from build123d import *

# Parameters (mm, degrees)
SZKIC1_R                    = 10.570763761
SZKIC1_R_2                  = 3
SZKIC1_R_3                  = 4
SZKIC1_R_4                  = 1
DODANIE_WYCI_GNI_CIE1_DEPTH = 5
SZKIC1_3_R                  = 10.570763761
SZKIC1_3_R_2                = 4
SZKIC1_3_R_3                = 1
DODANIE_WYCI_GNI_CIE2_DEPTH = 10


with BuildPart() as part:
    # Szkic1 → Dodanie-wyci_gni_cie1 (new body)
    with BuildSketch(Plane.XY):
        with BuildLine():
            Line((-50.67287635, -5.055665151), (-9.235111676, -10.570763761))
            ThreePointArc((-9.235111676, -10.570763761), (0, -11.182632843), (9.235111676, -10.570763761))
            Line((9.235111676, -10.570763761), (50.67287635, -5.055665151))
            ThreePointArc((50.67287635, -5.055665151), (55.100246338, 0), (50.67287635, 5.055665151))
            Line((50.67287635, 5.055665151), (9.235111676, 10.570763761))
            ThreePointArc((9.235111676, 10.570763761), (0, 11.182632843), (-9.235111676, 10.570763761))
            Line((-9.235111676, 10.570763761), (-50.67287635, 5.055665151))
            ThreePointArc((-50.67287635, 5.055665151), (-55.100246338, 0), (-50.67287635, -5.055665151))
        make_face()
        Circle(SZKIC1_R, mode=Mode.SUBTRACT)
        with Locations((50, 0)):
            Circle(SZKIC1_R_2, mode=Mode.SUBTRACT)
        with Locations((-50, 0)):
            Circle(SZKIC1_R_2, mode=Mode.SUBTRACT)
        Circle(SZKIC1_R)
        Circle(SZKIC1_R_3, mode=Mode.SUBTRACT)
        with Locations((-5.656854249, 5.656854249)):
            Circle(SZKIC1_R_4, mode=Mode.SUBTRACT)
        with Locations((-8, 0)):
            Circle(SZKIC1_R_4, mode=Mode.SUBTRACT)
        with Locations((0, 8)):
            Circle(SZKIC1_R_4, mode=Mode.SUBTRACT)
        with Locations((5.656854249, 5.656854249)):
            Circle(SZKIC1_R_4, mode=Mode.SUBTRACT)
        with Locations((8, 0)):
            Circle(SZKIC1_R_4, mode=Mode.SUBTRACT)
        with Locations((5.656854249, -5.656854249)):
            Circle(SZKIC1_R_4, mode=Mode.SUBTRACT)
        with Locations((0, -8)):
            Circle(SZKIC1_R_4, mode=Mode.SUBTRACT)
        with Locations((-5.656854249, -5.656854249)):
            Circle(SZKIC1_R_4, mode=Mode.SUBTRACT)
    extrude(amount=DODANIE_WYCI_GNI_CIE1_DEPTH)

    # Szkic1_3 → Dodanie-wyci_gni_cie2 (add)
    with BuildSketch(Plane.XY):
        Circle(SZKIC1_3_R)
        Circle(SZKIC1_3_R_2, mode=Mode.SUBTRACT)
        with Locations((-5.656854249, 5.656854249)):
            Circle(SZKIC1_3_R_3, mode=Mode.SUBTRACT)
        with Locations((-8, 0)):
            Circle(SZKIC1_3_R_3, mode=Mode.SUBTRACT)
        with Locations((0, 8)):
            Circle(SZKIC1_3_R_3, mode=Mode.SUBTRACT)
        with Locations((5.656854249, 5.656854249)):
            Circle(SZKIC1_3_R_3, mode=Mode.SUBTRACT)
        with Locations((8, 0)):
            Circle(SZKIC1_3_R_3, mode=Mode.SUBTRACT)
        with Locations((5.656854249, -5.656854249)):
            Circle(SZKIC1_3_R_3, mode=Mode.SUBTRACT)
        with Locations((0, -8)):
            Circle(SZKIC1_3_R_3, mode=Mode.SUBTRACT)
        with Locations((-5.656854249, -5.656854249)):
            Circle(SZKIC1_3_R_3, mode=Mode.SUBTRACT)
    extrude(amount=DODANIE_WYCI_GNI_CIE2_DEPTH)


solid = part.part
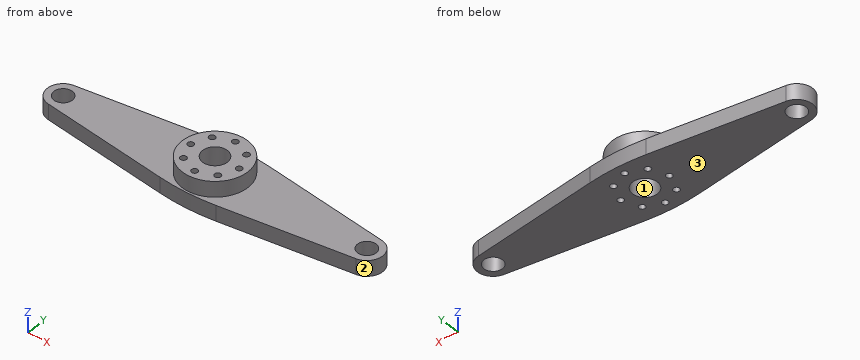
Geometry check sheet. Reference: the model listing, model coordinates, mm. Face numbers are marked on the shaded views. Round coordinates to 2 decimals unless told otherwise and drop trailing zeros. Order: outer loops, then holes, each group sorted by start corner. A loop starts at its lowest first (then second) coordinate and runs counter-clockwise, first axis right, second up. Notation, with made-up numbers: M 88,2 L 109,2 A27 cw 109,20 Z; hole C 19.5,-39 d11. An arc over 180 degrees is marked long. Write each question's results on one line, items separated by ' | '. Start each with the question number.
1. Cross-section at C-C on z = 6. Give the number of separate pieces and of enclosed holes in the cut face, plus the area to 3 significant figures.
2. Go/stop test with flat-tipped pins: P1, Ø10, axis at x = 26.5, y = -6.5, coming from the +Z side; P2, Ø6.5, axis at x = 0, y = 0, coming from the -Z side; P3, Ø2, axis at y = -2.5, z = 2, coming from the +X side; P4, Ø4, axis at y = 5, z = 8.5, coming from the +X side. Record where each tip stops, or that it passes through.
3. Draft check along X on the marked faces 1, 2 and 3. Enter one of: pulls with the +X half, pulls with the -X half, needs draft (parallel to the pull), parting line crosses it, or undercut.
4. Cross-section at B-B on y = -8. Record the boundary of the cut face in (x, z).
5. Cross-section at A-A on x = 0. Record the boundary of the cut face in (y, z), plus the area to 3 significant figures.
6. Material ranges on L1, parallel to Y at x = 0, z = 6.25; L2, parallel to X at y = 2, z = 2.5; L3, parallel to Z at x = -35, y = -6.75, recorded low to high. Write a range as from..to.
7. Cross-section at D-D on x = 43.5. Record the boundary of the cut face in (y, z), plus the area to 3 significant figures.
Resolved:
1) separate pieces: 1 | enclosed holes: 9 | area: 276 mm2
2) P1: z = 5 | P2: through | P3: x = 54.87 | P4: x = 10.14
3) face 1: undercut | face 2: pulls with the +X half | face 3: needs draft
4) outline: M -28.55,0 L -1,0 L -1,10 L -6.91,10 L -6.91,5 L -28.55,5 Z; M 1,0 L 28.55,0 L 28.55,5 L 6.91,5 L 6.91,10 L 1,10 Z
5) outline: M -11.18,0 L -9,0 L -9,10 L -10.57,10 L -10.57,5 L -11.18,5 Z; M -7,0 L -4,0 L -4,10 L -7,10 Z; M 4,0 L 7,0 L 7,10 L 4,10 Z; M 9,0 L 11.18,0 L 11.18,5 L 10.57,5 L 10.57,10 L 9,10 Z | area: 97.5 mm2
6) L1: -10.57..-9, -7..-4, 4..7, 9..10.57 | L2: -54.69..-52.24, -47.76..-3.46, 3.46..47.76, 52.24..54.69 | L3: 0..5
7) outline: M -6.01,0 L 6.01,0 L 6.01,5 L -6.01,5 Z | area: 60.1 mm2
